from build123d import *

# Parameters (mm, degrees)
F0_W     = 25.4
F0_H     = 25.4
F1_DEPTH = 25.4
F3_D     = 6.35
F3_DEPTH = 12.7
F3_TIP   = 1.9077324654


with BuildPart() as f1:
    # F0 (on Front) → F1 (new body)
    with BuildSketch(Plane.XZ):
        with Locations((12.7, 12.7)):
            Rectangle(F0_W, F0_H)
    extrude(amount=F1_DEPTH)

    # F3
    with Locations(Plane.XZ.offset(25.4)):
        with Locations((12.7, 12.7)):
            Hole(F3_D / 2, depth=F3_DEPTH)
            with Locations((0, 0, -(F3_DEPTH + F3_TIP / 2))):  # 118° drill point
                Cone(0, F3_D / 2, F3_TIP, mode=Mode.SUBTRACT)


solid = f1.part
Could you check a few things on this model? Use its own coordinates, in mm. Round coordinates to 2 decimals unless told otherwise and drop trailing zeros. Order: outer loops, then holes, each group sorted by start corner. A loop starts at its lowest first (then second) coordinate and runs counter-clockwise, first axis right, second up.
Q1. Imagine slicing it at A-A, the plane y = -18.5. List the corners of the cut face in (x, z) for me (3 decimals).
Geometry says:
outline: (0, 0) - (25.4, 0) - (25.4, 25.4) - (0, 25.4) - close; hole circle Ø6.35 at (12.7, 12.7)
Q2. Please list where these lines run through material, in increasing order: probe 1 along Z at (x, y) = (12.7, -18.5) (3 decimals); probe 2 along X at (y, z) = (-22, 12).
Geometry says:
probe 1: z = 0 to 9.525, 15.875 to 25.4
probe 2: x = 0 to 9.6, 15.8 to 25.4
Q3. Thinking about a two-plate mould opening in Z: for faces 1 (the face through (11.2, -19, 9.9)), 2 (the face through (13, -13, 25.4)), 3 (the face through (12.6, -11.1, 12.2)), 4 (the face through (13, 0, 13)), which applies, released by +Z, released by -Z, zero draft, split by the parting line, or undercut?
Geometry says:
face 1: undercut
face 2: released by +Z
face 3: undercut
face 4: zero draft
